from build123d import *

# Parameters (mm, degrees)
CROQUIS1_W              = 170
CROQUIS1_H              = 50.8
CROQUIS1_R              = 10
SALIENTE_EXTRUIR1_DEPTH = 12.7
CROQUIS2_R              = 2.5
CORTAR_EXTRUIR1_DEPTH   = 32.7
CROQUIS3_R              = 2.5
CORTAR_EXTRUIR2_DEPTH   = 40


with BuildPart() as part:
    # Croquis1 → Saliente-Extruir1 (new body)
    with BuildSketch(Plane.XY):
        Rectangle(CROQUIS1_W, CROQUIS1_H)
        with Locations((52.5, 5)):
            Circle(CROQUIS1_R, mode=Mode.SUBTRACT)
        with Locations((-52.5, 5)):
            Circle(CROQUIS1_R, mode=Mode.SUBTRACT)
    extrude(amount=SALIENTE_EXTRUIR1_DEPTH)

    # Croquis2 → Cortar-Extruir1 (cut)
    with BuildSketch(Plane.XZ.offset(25.4)):
        with Locations((-52.5, 6.35)):
            Circle(CROQUIS2_R)
        with Locations((52.5, 6.35)):
            Circle(CROQUIS2_R)
    extrude(amount=-CORTAR_EXTRUIR1_DEPTH, mode=Mode.SUBTRACT)

    # Croquis3 → Cortar-Extruir2 (cut)
    with BuildSketch(Plane.XZ.offset(25.4)):
        with Locations((-73, 6.35)):
            Circle(CROQUIS3_R)
        with Locations(Location((73, 6.35, 0), (0, 0, 180))):
            Circle(CROQUIS3_R)
    extrude(amount=-CORTAR_EXTRUIR2_DEPTH, mode=Mode.SUBTRACT)


solid = part.part
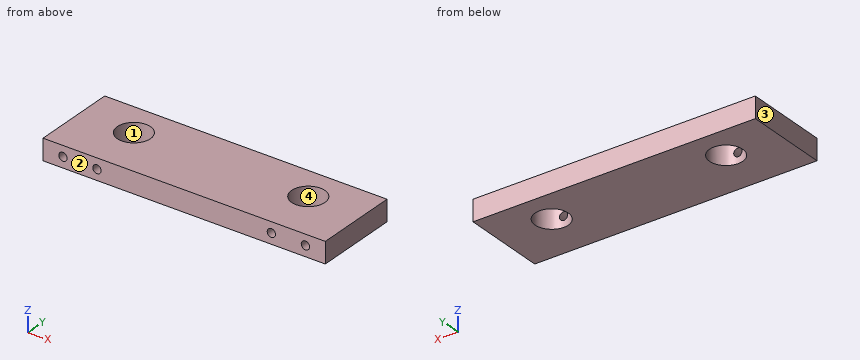
Work out the finished part from the listing and answer in its coordinate system (mm). Face numbers are marked on the shaded views. Coordinates: 2 decimals unless noted, no trailing zeros. Write each loop counter-clockwise with the first axis right and the second up, starting at its lowest first coordinate (ties: lowest second). Pieces come first, ordered by that corner, then holes. Notation, with made-up numbers: M 47.5,-12.75 L 96.5,-12.75 A11 ccw 96.5,1.25 Z; hole C 25.25,10.5 d8. An arc over 180 degrees is marked long. Answer as CSV lines item,"result". Start each with the question number.
Item 1: Section A-A on y = 5 is taken. Write down the section's boundary in (x, z), and give its area (3 significant figures).
Item 2: Section C-C on x = 52.5 is taken. Write down the section's boundary in (y, z), and give its area (3 significant figures).
Item 3: Consider L1, parallel to Z at x = -73, y = -16; L2, parallel to X at y = 13, z = 5.75; L3, parallel to X at y = 8, z = 6. Determine where each line is inside the solid, lowest interval first.
Item 4: Flat-ended cylindrical pins translate along their axes: P1, Ø1.5, axis at x = -73, z = 6.5, coming from the -Y side; P2, Ø2, axis at x = -59, y = 1.5, coming from the -Z side. Find the tip coordinate at first contact, or state that the pin passes through.
Item 5: Determine the mould class of the marked faces 1, 2, 3 and 4 for opening direction Y: released by +Y, released by -Y, zero draft, split by the parting line, or undercut.
Item 6: Section B-B on z = 6.35 is taken. Write down the section's boundary in (x, y), and give its area (3 significant figures).
Item 7: Section D-D on y = -16 is taken. Write down the section's boundary in (x, z), and give its area (3 significant figures).
Checks:
1,outline,"M -85,0 L -62.5,0 L -62.5,12.7 L -85,12.7 Z; M -42.5,0 L 42.5,0 L 42.5,12.7 L -42.5,12.7 Z; M 62.5,0 L 85,0 L 85,12.7 L 62.5,12.7 Z; hole C -73,6.35 d5; hole C 73,6.35 d5"
1,area,"1,610 mm²"
2,outline,"M -25.4,0 L -5,0 L -5,3.85 L -25.4,3.85 Z; M -25.4,8.85 L -5,8.85 L -5,12.7 L -25.4,12.7 Z; M 15,0 L 25.4,0 L 25.4,12.7 L 15,12.7 Z"
2,area,"289 mm²"
3,L1,"z = 0 to 3.85, 8.85 to 12.7"
3,L2,"x = -85 to -75.43, -70.57 to -58.5, -46.5 to 46.5, 58.5 to 70.57, 75.43 to 85"
3,L3,"x = -85 to -75.48, -70.52 to -62.04, -42.96 to 42.96, 62.04 to 70.52, 75.48 to 85"
4,P1,"stops at y = 14.6"
4,P2,"passes through"
5,face 1,"undercut"
5,face 2,"released by -Y"
5,face 3,"zero draft"
5,face 4,"undercut"
6,outline,"M -85,-25.4 L -75.5,-25.4 L -75.5,14.6 L -70.5,14.6 L -70.5,-25.4 L -55,-25.4 L -55,-4.68 A10 cw long -50,-4.68 L -50,-25.4 L 50,-25.4 L 50,-4.68 A10 cw long 55,-4.68 L 55,-25.4 L 70.5,-25.4 L 70.5,14.6 L 75.5,14.6 L 75.5,-25.4 L 85,-25.4 L 85,25.4 L -85,25.4 Z"
6,area,"7,400 mm²"
7,outline,"M -85,0 L 85,0 L 85,12.7 L -85,12.7 Z; hole C -73,6.35 d5; hole C -52.5,6.35 d5; hole C 52.5,6.35 d5; hole C 73,6.35 d5"
7,area,"2,080 mm²"
